Can you work these out from the model? Positions are in its coordinate system, mm. Round coordinates to 2 decimals unless told otherwise and drop trailing zeros. Loops run counter-clockwise (first coordinate to the right, second up) from the corner with the lowest first, then second, coordinate; pieces in that order, holes last. Notation, with made-up numbers: (65, 58.25) -> (74, 58.25) arc R26 ccw to (74, 81.25) -> close; hole circle Ø8 at (54.5, -1). An arc over 180 degrees is marked (long way). Write each question's results on one line, items separated by ' | '.
from build123d import *

# Parameters (mm, degrees)
F1_DEPTH = 3
F2_R     = 3
F3_DEPTH = 25.4
F4_R     = 3
F5_DEPTH = 25


with BuildPart() as f1:
    # F0 (on Front) → F1 (new body)
    with BuildSketch(Plane.XZ):
        with BuildLine():
            ThreePointArc((-10, 80), (0, 70), (10, 80))
            ThreePointArc((10, 80), (0, 90), (-10, 80))
        make_face()
        with BuildLine():
            Line((10, -60), (10, 80))
            ThreePointArc((10, 80), (0, 70), (-10, 80))
            Line((-10, 80), (-10, -60))
            ThreePointArc((-10, -60), (0, -50), (10, -60))
        make_face()
        with BuildLine():
            ThreePointArc((-10, -60), (0, -70), (10, -60))
            ThreePointArc((10, -60), (0, -50), (-10, -60))
        make_face()
    extrude(amount=F1_DEPTH)

    # F2 (on face) → F3 (cut)
    with BuildSketch(Plane.XZ.offset(3)):
        with Locations((0, 80)):
            Circle(F2_R)
        with Locations((0, -60)):
            Circle(F2_R)
    extrude(amount=-F3_DEPTH, mode=Mode.SUBTRACT)

    # F4 (on face) → F5 (cut)
    with BuildSketch(Plane.XZ.offset(3)):
        with Locations((0, 17)):
            Circle(F4_R)
    extrude(amount=-F5_DEPTH, mode=Mode.SUBTRACT)


solid = f1.part
1. Please list where these lines run through material, in increasing order: line 1 (Z direction, x = 0, y = -0.9); line 2 (Z direction, x = -2, y = -0.8); line 3 (X direction, y = -2.1, z = 82). Write a range as from..to.
Final values:
line 1: -70..-63, -57..14, 20..77, 83..90 | line 2: -69.8..-62.24, -57.76..14.76, 19.24..77.76, 82.24..89.8 | line 3: -9.8..-2.24, 2.24..9.8
2. Will these pins go through, and if not, where does the flat tip stop? pin 1 (5.5 mm diameter, centred on x = 0, z = 17, fed in from -Y); pin 2 (9.5 mm diameter, centred on x = 0, z = -60, fed in from -Y).
Final values:
pin 1: through | pin 2: y = -3
3. If we section it at A-A (z = 17): List the corners of the cut face in (x, y) for me, then the cut area to 3 significant figures.
Final values:
outline: (-10, -3) -> (-3, -3) -> (-3, 0) -> (-10, 0) -> close; (3, -3) -> (10, -3) -> (10, 0) -> (3, 0) -> close | area: 42.0 mm2
4. If we section it at B-B (y = -1.1): List the corners of the cut face in (x, z) for me.
Final values:
outline: (-10, -60) arc R10 ccw to (10, -60) -> (10, 80) arc R10 ccw to (-10, 80) -> close; hole circle Ø6 at (0, -60); hole circle Ø6 at (0, 17); hole circle Ø6 at (0, 80)
5. If we section it at D-D (x = 8): List the corners of the cut face in (y, z) for me, then the cut area to 3 significant figures.
Final values:
outline: (-3, -66) -> (0, -66) -> (0, 86) -> (-3, 86) -> close | area: 456 mm2
6. We'd pull the mould along Z, two halves only. Please class faces 1 (the face through (0, -1, -70)), 2 (the face through (0, -2, -57)), 3 (the face through (0, -3, 11)), 4 (the face through (-0.65, -1.52, 77.07)): pulls with the +Z half, pulls with the -Z half, needs draft (parallel to the pull), parting line crosses it, or undercut.
Final values:
face 1: pulls with the -Z half | face 2: undercut | face 3: needs draft | face 4: undercut
7. If we section it at C-C (x = 1): List the corners of the cut face in (y, z) for me.
Final values:
outline: (-3, -69.95) -> (0, -69.95) -> (0, -62.83) -> (-3, -62.83) -> close; (-3, -57.17) -> (0, -57.17) -> (0, 14.17) -> (-3, 14.17) -> close; (-3, 19.83) -> (0, 19.83) -> (0, 77.17) -> (-3, 77.17) -> close; (-3, 82.83) -> (0, 82.83) -> (0, 89.95) -> (-3, 89.95) -> close
